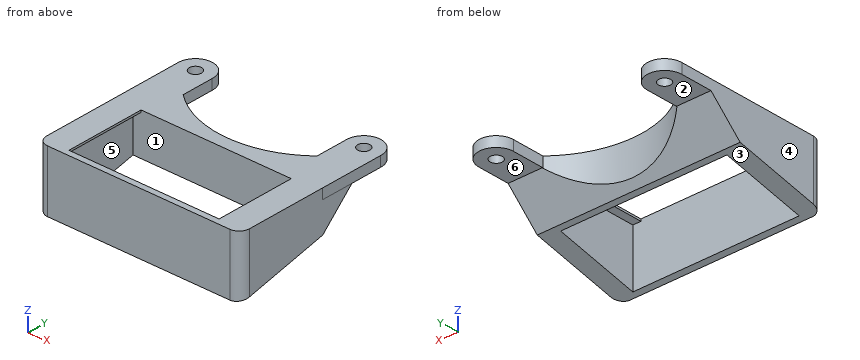
from build123d import *

# Parameters (mm, degrees)
F0_W      = 100
F0_H      = 45
F1_DEPTH  = 30
F2_W      = 74
F2_H      = 39.3
F3_DEPTH  = 30.001
F5_DEPTH  = 100.001
F7_DEPTH  = 5
F10_DEPTH = 100
F12_DEPTH = 25.4
F13_R     = 3
F14_DEPTH = 25.4
F15_R     = 5.08
F17_DEPTH = 4
F19_DEPTH = 4


with BuildPart() as f1:
    # F0 (on Top) → F1 (new body)
    with BuildSketch(Plane.XY):
        with Locations((50, 22.5)):
            Rectangle(F0_W, F0_H)
    extrude(amount=F1_DEPTH)

    # F2 (on face) → F3 (cut, through all)
    with BuildSketch(Plane.XY.offset(30)):
        with Locations((50, 22.55)):
            Rectangle(F2_W, F2_H)
    extrude(amount=-F3_DEPTH, mode=Mode.SUBTRACT)

    # F4 (on face) → F5 (cut, through all)
    with BuildSketch(Plane(origin=(0, 0, 0), x_dir=(0, -1, 0), z_dir=(-1, 0, 0))):
        Polygon((-45, 0), (0, 0), (-45, 10), align=None)
    extrude(amount=-F5_DEPTH, mode=Mode.SUBTRACT)

    # F6 (on face) → F7 (join)
    with BuildSketch(Plane.XY.offset(30)):
        with BuildLine():
            Line((16.9887500545, 60.6564121963), (16.9887500545, 76.3128243926))
            ThreePointArc((16.9887500545, 76.3128243926), (8.7186601661, 85.2471870482), (0, 76.75))
            Line((0, 76.75), (0, 45))
            Line((0, 45), (100, 45))
            Line((100, 45), (99.9984056515, 76.5853750228))
            ThreePointArc((99.9984056515, 76.5853750228), (91.5120769432, 85.2499914204), (83.0011608569, 76.609525019))
            Line((83.0011608569, 76.609525019), (83.0011608569, 60.6564121963))
            Line((83.0011608569, 60.6564121963), (16.9887500545, 60.6564121963))
        make_face()
    extrude(amount=-F7_DEPTH)

    # F8: union 

    # F9 (on face) → F10 (join)
    with BuildSketch(Plane(origin=(0, 0, 0), x_dir=(0, -1, 0), z_dir=(-1, 0, 0))):
        Polygon((-60.875, 25), (-45, 10), (-45, 25), align=None)
    extrude(amount=-F10_DEPTH)

    # F11 (on face) → F12 (cut)
    with BuildSketch(Plane.XY.offset(30)):
        with BuildLine():
            Line((16.9887500545, 65.0414451957), (16.9887500545, 60.6564121963))
            ThreePointArc((16.9887500545, 60.6564121963), (49.9949554557, 48.3478851896), (83.0011608569, 60.6564121963))
            Line((83.0011608569, 60.6564121963), (83.0011608569, 65.0414451957))
            Line((83.0011608569, 65.0414451957), (16.9887500545, 65.0414451957))
        make_face()
    extrude(amount=-F12_DEPTH, mode=Mode.SUBTRACT)

    # F13 (on face) → F14 (cut)
    with BuildSketch(Plane.XY.offset(30)):
        with Locations((8.5, 76.75)):
            Circle(F13_R)
        with Locations((91.5, 76.75)):
            Circle(F13_R)
    extrude(amount=-F14_DEPTH, mode=Mode.SUBTRACT)

    # F15
    f15_edges = [f1.edges().sort_by_distance(p)[0] for p in [
        (0, 0, 15),
        (100, 0, 15),
    ]]
    fillet(f15_edges, radius=F15_R)

    # F16 (on face) → F17 (cut)
    with BuildSketch(Plane.YZ.offset(13)):
        Polygon((2.9, 29), (2.9, 0.6444444444), (42.2, 9.3777777778), (42.2, 29), align=None)
    extrude(amount=-F17_DEPTH, mode=Mode.SUBTRACT)

    # F18 (on face) → F19 (cut)
    with BuildSketch(Plane(origin=(87, 0, 0), x_dir=(0, -1, 0), z_dir=(-1, 0, 0))):
        Polygon((-42.2, 9.3777777778), (-2.9, 0.6444444444), (-2.9, 29), (-42.2, 29), align=None)
    extrude(amount=-F19_DEPTH, mode=Mode.SUBTRACT)


solid = f1.part
Work out the finished part from the listing and answer in its coordinate system (mm). Face numbers are marked on the shaded views. A direction names the side the tool comes from. Coordinates: 2 decimals unless noted, no trailing zeros. Loops run counter-clockwise (first coordinate to the right, second up) from the corner with the lowest first, then second, coordinate; pieces in that order, holes last. Notation, with made-up numbers: M -16,-32.5 L 14,-32.5 A9 ccw 14,-27.5 Z; hole C 63.25,-0.5 d7. An arc over 180 degrees is marked long. Answer in a Markdown table with one row per item. Add a question column.
1. Flat-ended cylindrical pins translate along their axes: P1, Ø13.5, axis at x = 9, y = 77, coming from the -Z side; P2, Ø4, axis at x = 16.5, y = 15.5, coming from the -Z side; P3, Ø7, axis at x = 91.5, y = 76.75, coming from the +Z side; P4, Ø4.5, axis at x = 10.5, y = 25, coming from the -Z side. Find the tip coordinate at first contact, or state that the pin passes through.
2. Find section C-C, the plane z = 27.75. Write down the section's boundary in (x, y).
3. Consider L1, parallel to Y at x = 8.5, z = 26.8; L2, parallel to X at y = 40, z = 14.5; L3, parallel to Z at x = 89.5, y = 21. Determine where each line is inside the solid, lowest interval first.
4. Find section B-B, the plane x = 39. Write down the section's boundary in (y, z), then the cut area to 3 significant figures.
5. Find section D-D, the plane y = 41. Write down the section's boundary in (x, z).
6. The mould has two halves that part along Y. Classify the marked faces 1, 2 and 3: pulls with the +Y half, pulls with the -Y half, needs draft (parallel to the pull), parting line crosses it, or undercut.
7. Find section A-A, the plane y = 9. Write down the section's boundary in (x, z), then the cut area to 3 significant figures.
8. A tool of negligible diameter and unlimited length cuts with its end or side. For the marked faces 4, 5 and 6, from which of +Z, -Z, +X, -X, +Y, -Y can it reach the whole face along a straight path? Write none if from no direction.
Reported:
| question | item | result |
|---|---|---|
| 1 | P1 | stops at z = 25 |
| 1 | P2 | passes through |
| 1 | P3 | stops at z = 30 |
| 1 | P4 | stops at z = 5.18 |
| 2 | outline | M 0,5.08 A5.08 ccw 5.08,0 L 94.92,0 A5.08 ccw 100,5.08 L 100,45 L 100,76.59 A8.5 ccw long 83,76.61 L 83,60.66 A50.41 cw 16.99,60.66 L 16.99,76.31 A8.5 ccw long 0,76.75 Z; hole C 8.5,76.75 d6; hole M 9,2.9 L 91,2.9 L 91,42.2 L 9,42.2 Z; hole C 91.5,76.75 d6 |
| 3 | L1 | y = 0 to 73.75, 79.75 to 85.25 |
| 3 | L2 | x = 0 to 9, 91 to 100 |
| 3 | L3 | z = 29 to 30 |
| 4 | outline | M 0,0 L 2.9,0.64 L 2.9,30 L 0,30 Z; M 42.2,9.38 L 45,10 L 49.56,14.31 L 49.56,30 L 42.2,30 Z |
| 4 | area | 224 mm^2 |
| 5 | outline | M 0,9.11 L 9,9.11 L 9,29 L 13,29 L 13,30 L 0,30 Z; M 87,29 L 91,29 L 91,9.11 L 100,9.11 L 100,30 L 87,30 Z |
| 6 | face 1 | undercut |
| 6 | face 2 | needs draft |
| 6 | face 3 | pulls with the +Y half |
| 7 | outline | M 0,2 L 9,2 L 9,29 L 13,29 L 13,30 L 0,30 Z; M 87,29 L 91,29 L 91,2 L 100,2 L 100,30 L 87,30 Z |
| 7 | area | 512 mm^2 |
| 8 | face 4 | +Z, -Z, -X, +Y, -Y |
| 8 | face 5 | -Z |
| 8 | face 6 | -Z, +X, -X, +Y |
